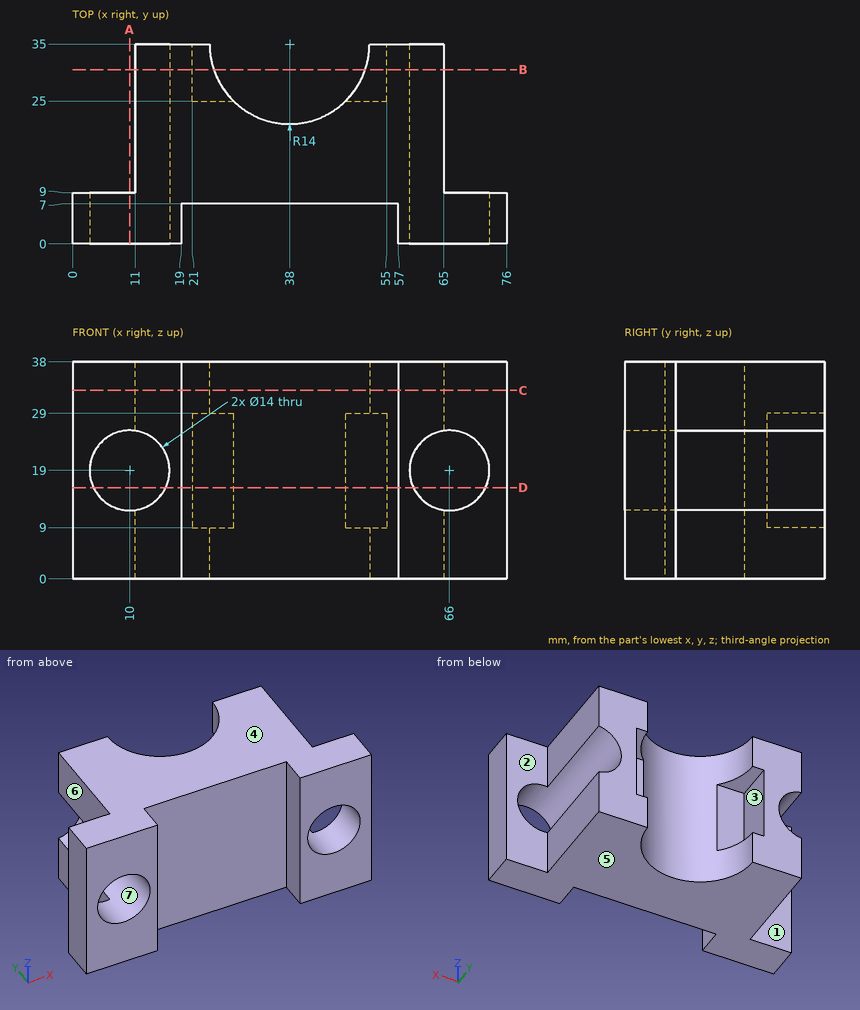
The figure shows three views and two pictorial views of one solid part (mm, origin at its lowest corner). Answer the questions. A direction names the side the tool comes from. Round coordinates to 2 decimals unless told otherwise and drop trailing zeros. Write each loop counter-clockwise with the first axis right and the second up, starting at its lowest first coordinate (ties: lowest second). Pieces come first, ordered by that corner, then holes. Notation, with made-up numbers: (-40, -35.75) - (-13, -35.75) arc R34 ccw to (-13, -0.75) - close; hole circle Ø3 at (40, 2). An arc over 180 degrees is marked (long way). Answer in a Markdown table with one row per item. Add a question column.
1. A cutting plane is placed at A-A, the plane x = 10. Determine the outline of the cut face in (y, z).
2. A cutting plane is placed at B-B, the plane y = 30.5. Determine the outline of the cut face in (x, z).
3. A cutting plane is placed at D-D, the plane z = 16. Determine the outline of the cut face in (x, y), and give its area (3 significant figures).
4. For the marked faces 1, 2 and 3, determine the directions among +Z, -Z, +X, -X, +Y, -Y from which every point of the face is accessible in a straight line to the end or side of a thin tool.
5. Given pin 1 (6 mm diameter, centred on y = 21, z = 7.5, fed in from +X); pin 2 (8 mm diameter, centred on x = 26, z = 14.5, fed in from +Y); pin 3 (4 mm diameter, centred on x = 31.5, z = 22, fed in from +Y), each flat-ended and moving along its own axis, determine where each tip first touches the part or whether it passes through.
6. Find the intervals of material crossed by line 1 along X through (y, z) = (8, 19); line 2 along Z through (x, y) = (10, 7); line 3 along X through (y, z) = (28, 19), in increasing order. Write a range as from..to.
7. A cutting plane is placed at C-C, the plane z = 33. Determine the outline of the cut face in (x, y), and give its area (3 significant figures).
8. The mould has two halves that part along Z. Classify the marked faces 4, 5, 6 and 7: +Z half, -Z half, draft (parallel to the pull), parting line (faces both ways), or undercut.
Worked out:
| question | item | result |
|---|---|---|
| 1 | outline | (0, 0) - (9, 0) - (9, 12) - (0, 12) - close; (0, 26) - (9, 26) - (9, 38) - (0, 38) - close |
| 2 | outline | (11, 0) - (24.74, 0) - (24.74, 9) - (21, 9) - (21, 29) - (24.74, 29) - (24.74, 38) - (11, 38) - (11, 25.93) arc R7 cw to (11, 12.07) - close; (51.26, 0) - (65, 0) - (65, 12.07) arc R7 cw to (65, 25.93) - (65, 38) - (51.26, 38) - (51.26, 29) - (55, 29) - (55, 9) - (51.26, 9) - close |
| 3 | outline | (0, 0) - (3.68, 0) - (3.68, 9) - (0, 9) - close; (16.32, 0) - (19, 0) - (19, 7) - (57, 7) - (57, 0) - (59.68, 0) - (59.68, 35) - (55, 35) - (55, 25) - (47.8, 25) arc R14 cw to (28.2, 25) - (21, 25) - (21, 35) - (16.32, 35) - close; (72.32, 0) - (76, 0) - (76, 9) - (72.32, 9) - close |
| 3 | area | 923 mm^2 |
| 4 | face 1 | +Z, -Z, -X, +Y |
| 4 | face 2 | +Z, -Z, +X, +Y |
| 4 | face 3 | +Y |
| 5 | pin 1 | x = 65 |
| 5 | pin 2 | y = 25 |
| 5 | pin 3 | y = 23.88 |
| 6 | line 1 | 0..3, 17..59, 73..76 |
| 6 | line 2 | 0..12, 26..38 |
| 6 | line 3 | 17..21, 55..59 |
| 7 | outline | (0, 0) - (19, 0) - (19, 7) - (57, 7) - (57, 0) - (76, 0) - (76, 9) - (65, 9) - (65, 35) - (52, 35) arc R14 cw to (24, 35) - (11, 35) - (11, 9) - (0, 9) - close |
| 7 | area | 1,510 mm^2 |
| 8 | face 4 | +Z half |
| 8 | face 5 | -Z half |
| 8 | face 6 | draft |
| 8 | face 7 | undercut |
